Design review of the part built by this model. Coordinates are the model's own, in mm. A direction names the side the tool comes from. Round coordinates to 2 decimals unless told otherwise and drop trailing zeros. Write each loop counter-clockwise with the first axis right and the second up, starting at its lowest first coordinate (ties: lowest second). Pieces come first, ordered by that corner, then holes. Notation, with made-up numbers: (-21.75, 63) -> (29.25, 63) arc R10 ccw to (29.25, 76) -> close; hole circle Ø4 at (-38, 80). An arc over 180 degrees is marked (long way). Write item = value, one per line. Start each with the question number.
Item 1: Machinability: for faces 5 (the flat face through (-18.02, -1.97, -5.53)), 6 (the cylindrical face through (-11.48, -0.57, -18.59)), 7 (the flat face through (-17, -10, -9)), 8 (the flat face through (-28, 0, -7.5)), 9 (the cylindrical face through (-13.4, -5, -16)), which of the approach directions +Z, -Z, +X, -X, +Y, -Y give a long, thin tool a straight path to every point of the face, cutting with its end or side? Answer none if there is none.
Item 2: Add section A-A, the plane x = -21.5. State the section outline as (y, z) points, then the cut area to 3 significant figures.
Item 3: Mouldability with a two-part tool opening along Z and no side actions: class faces 1 (the cylindrical face through (-13.3, 5, -16)), 2 (the flat face through (-21, -3, -3.5)), 3 (the flat face through (-19, 2, 0)), 4 (the flat face through (-19, 6, -13)) as released by +Z, released by -Z, zero draft, split by the parting line, or undercut.
Item 4: Add section B-B, the plane z = -16. State the section outline as (x, y) points, then the cut area to 3 significant figures.
Item 5: For pin 1 Ø3 at (y, z) = (4, -15.5) entering from -X; pin 2 Ø5 at (y, z) = (7, -20.5) entering from +X; pin 3 Ø5 at (x, y) = (-21.5, 0) entering from +Z; pin 4 Ø1.9 at (x, y) = (-26, 0.5) entering from -Z, all flat-tipped, find the tip position at first contact; note any pin that passes through.
Item 6: Add section D-D, the plane y = -1.25. State the section outline as (x, z) points.
Item 7: Add section C-C, the plane x = -11.5. State the section outline as (y, z) points, then the cut area to 3 significant figures.
Item 8: To check wall thickness, follow L1, parallel to Y at x = -21.5, z = -2.45; L2, parallel to X at y = 0, z = -1.9; L3, parallel to Y at x = -21, z = -6.5. State the ranges of each line that lie inside material, in increasing order.
from build123d import *

# Parameters (mm, degrees)
F0_W      = 2
F0_H      = 4.5
F1_DEPTH  = 7.5
F3_DEPTH  = 10
F5_DEPTH  = 6
F6_SIZE   = 2
F7_SIZE   = 2
F8_R      = 2.65
F9_DEPTH  = 25
F10_SIZE  = 2
F11_R     = 5
F12_DEPTH = 25
F13_W     = 22
F13_H     = 24.5
F14_DEPTH = 25
F16_DEPTH = 4
F17_R     = 2.75
F18_DEPTH = 25


with BuildPart() as f1:
    # F0 (on Top) → F1 (new body, symmetric)
    with BuildSketch(Plane.XY):
        with Locations((-9, 0)):
            Rectangle(F0_W, F0_H)
    extrude(amount=F1_DEPTH, both=True)

    # F2 (on Front) → F3 (join, symmetric)
    with BuildSketch(Plane.XZ):
        Polygon((-10, -24.5), (-10, 24.5), (-13, 24.5), (-30, 7.5), (-30, -7.5), (-13, -24.5), align=None)
    extrude(amount=F3_DEPTH, both=True)

    # F4 (on Front) → F5 (cut, symmetric)
    with BuildSketch(Plane.XZ):
        Polygon((-13, 7.5), (-13, 24.5), (-30, 7.5), align=None)
        Polygon((-13, -7.5), (-30, -7.5), (-13, -24.5), align=None)
    extrude(amount=F5_DEPTH, both=True, mode=Mode.SUBTRACT)

    # F6
    f6_edges = [f1.edges().sort_by_distance(p)[0] for p in [
        (-13, 6, -16),
        (-21.5, 6, -7.5),
        (-13, 0, -7.5),
        (-21.5, -6, -7.5),
        (-13, -6, -16),
        (-21.5, -6, 7.5),
        (-13, -6, 16),
        (-13, 6, 16),
        (-21.5, 6, 7.5),
        (-13, 0, 7.5),
    ]]
    chamfer(f6_edges, length=F6_SIZE)

    # F7
    f7_edges = [f1.edges().sort_by_distance(p)[0] for p in [
        (-30, -10, 0),
        (-30, 10, 0),
    ]]
    chamfer(f7_edges, length=F7_SIZE)

    # F8 (on face) → F9 (cut)
    with BuildSketch(Plane.YZ.offset(-10)):
        with Locations((0, -16)):
            Circle(F8_R)
        with Locations((0, 16)):
            Circle(F8_R)
    extrude(amount=-F9_DEPTH, mode=Mode.SUBTRACT)

    # F10
    f10_edges = [f1.edges().sort_by_distance(p)[0] for p in [
        (-11.5, 10, -24.5),
        (-11.5, -10, -24.5),
        (-11.5, 10, 24.5),
        (-11.5, -10, 24.5),
    ]]
    chamfer(f10_edges, length=F10_SIZE)

    # F11 (on face) → F12 (cut)
    with BuildSketch(Plane(origin=(-13, 0, 0), x_dir=(0, -1, 0), z_dir=(-1, 0, 0))):
        with Locations((0, 16)):
            Circle(F11_R)
        with Locations((0, -16)):
            Circle(F11_R)
    extrude(amount=F12_DEPTH, mode=Mode.SUBTRACT)

    # F13 (on face) → F14 (cut)
    with BuildSketch(Plane.XZ.offset(10)):
        with Locations((-19, 12.25)):
            Rectangle(F13_W, F13_H)
    extrude(amount=-F14_DEPTH, mode=Mode.SUBTRACT)

    # F15 (on face) → F16 (cut)
    with BuildSketch(Plane(origin=(0, 0, -7.5), x_dir=(1, 0, 0), z_dir=(0, 0, -1))):
        Polygon((-19.190599, 4), (-23.809401, 4), (-26.118802, 0), (-23.809401, -4), (-19.190599, -4), (-16.881198, 0), align=None)
    extrude(amount=-F16_DEPTH, mode=Mode.SUBTRACT)

    # F17 (on face) → F18 (cut)
    with BuildSketch(Plane(origin=(0, 0, -3.5), x_dir=(1, 0, 0), z_dir=(0, 0, -1))):
        with Locations((-21.5, 0)):
            Circle(F17_R)
    extrude(amount=-F18_DEPTH, mode=Mode.SUBTRACT)


solid = f1.part
Result set:
q1.face_5 = -Z
q1.face_6 = +X, -X
q1.face_7 = +Z, -Z, +X, -X, -Y
q1.face_8 = -Z, -X
q1.face_9 = -X
q2.outline = (-10, -16) -> (-6, -16) -> (-6, -9.5) -> (-4, -7.5) -> (-4, -3.5) -> (-2.75, -3.5) -> (-2.75, 0) -> (-10, 0) -> close; (2.75, -3.5) -> (4, -3.5) -> (4, -7.5) -> (6, -9.5) -> (6, -16) -> (10, -16) -> (10, 0) -> (2.75, 0) -> close
q2.area = 171 mm²
q3.face_1 = undercut
q3.face_2 = released by -Z
q3.face_3 = released by +Z
q3.face_4 = zero draft
q4.outline = (-21.5, -10) -> (-10, -10) -> (-10, -2.65) -> (-13, -2.65) -> (-13, -5) -> (-14, -5) -> (-15, -6) -> (-21.5, -6) -> close; (-21.5, 6) -> (-15, 6) -> (-14, 5) -> (-13, 5) -> (-13, 2.65) -> (-10, 2.65) -> (-10, 10) -> (-21.5, 10) -> close
q4.area = 115 mm²
q5.pin_1 = -14.5
q5.pin_2 = -10
q5.pin_3 = through
q5.pin_4 = -7.5
q6.outline = (-30, -7.5) -> (-25.4, -7.5) -> (-25.4, -3.5) -> (-23.95, -3.5) -> (-23.95, 0) -> (-30, 0) -> close; (-19.05, -3.5) -> (-17.6, -3.5) -> (-17.6, -7.5) -> (-15, -7.5) -> (-13, -9.5) -> (-13, -13.66) -> (-10, -13.66) -> (-10, -7.5) -> (-8, -7.5) -> (-8, 0) -> (-19.05, 0) -> close; (-13, -24.5) -> (-10, -24.5) -> (-10, -18.34) -> (-13, -18.34) -> close
q7.outline = (-10, -22.5) -> (-8, -24.5) -> (8, -24.5) -> (10, -22.5) -> (10, 0) -> (-10, 0) -> close; hole circle Ø5.3 at (0, -16)
q7.area = 464 mm²
q8.L1 = -10 to -2.75, 2.75 to 10
q8.L2 = -30 to -24.25, -18.75 to -8
q8.L3 = -10 to -4, 4 to 10
